For this review, take the finished solid that the model builds, in its own axes (mm). A direction names the side the tool comes from. Coordinates: 2 decimals unless noted, no trailing zeros. Write each loop counter-clockwise with the first axis right and the second up, starting at its lowest first coordinate (ties: lowest second). Pieces come first, ordered by that corner, then holes.
1) Insertion check: P1, Ø5.5, axis at y = 8, z = 6.5, coming from the +X side; P2, Ø3, axis at x = 2, y = -10.5, coming from the -Z side; P3, Ø4, axis at x = 0.5, y = 6.5, coming from the -Z side; P4, Ø1.5, axis at y = 6, z = 8, coming from the -X side. Each pin has a flat end and moves straight along its axis. Give the tip position at first contact, or say it passes through.
2) Mouldability with a two-part tool opening along X and no side actions: class faces 1 (the face through (-1.35, -9, 9)), 2 (the face through (0.942, 2.272, 4.052)), 3 (the face through (0.02, -6.2, 10.37)), 4 (the face through (4.506, -0.082, 3.944)) as pulls with the +X half, pulls with the -X half, needs draft (parallel to the pull), parting line crosses it, or undercut.
3) To check wall thickness, follow line 1 along Y through (x, z) = (0, 2.25); line 2 along Y through (x, z) = (1, 10.75); line 3 along X through (y, z) = (8.5, 13). State the ranges of each line that lie inside material, in increasing order.
4) We need section D-D on z = 2.25. Write out the cut boundary in (x, y), then the cut area to 3 significant figures.
5) We need section A-A on y = 0. Write out the cut boundary in (x, z), then the cut area to 3 significant figures.
6) We need section C-C on z = 10.25. Write out the cut boundary in (x, y), then the cut area to 3 significant figures.
7) For faces 5 (the face through (-3, -1, 8)), 6 (the face through (-0.02, 13.49, 14.13)), list the 3-axis set-ups (+Z, -Z, +X, -X, +Y, -Y) from which the entire face can be reached by the end or side of a thin tool; tool diameter is ignored.
from build123d import *

# Parameters (mm, degrees)
PAD_DEPTH = 1.35


with BuildPart() as pad:
    # Sketch001 → Pad (new body, symmetric)
    with BuildSketch(Plane.YZ):
        with BuildLine():
            Line((3, 0), (3, 8))
            Line((3, 8), (5, 8))
            Line((5, 8), (7.430632, 12.805439))
            ThreePointArc((13.716382, 8.063801), (13.408875, 14.193324), (7.430632, 12.805439))
            Line((5, 0), (13.716382, 8.063801))
            Line((3, 0), (5, 0))
        make_face()
        with BuildLine():
            Line((-13.716382, 8.063801), (-5, 0))
            Line((-5, 0), (-3, 0))
            Line((-3, 0), (-3, 8))
            Line((-3, 8), (-5, 8))
            Line((-5, 8), (-7.430632, 12.805439))
            ThreePointArc((-7.430632, 12.805439), (-13.408875, 14.193324), (-13.716382, 8.063801))
        make_face()
    extrude(amount=PAD_DEPTH, both=True)


with BuildPart() as obj1:
    # Sketch → Revolution (revolve)
    with BuildSketch(Plane.YZ):
        Polygon((3, 0), (2.46, 0.311769), (2.46, 7.688231), (3, 8), (4, 8), (5, 0), align=None)
    revolve(axis=Axis((0, 0, 0), (0, 0, 1)))

    # Fusion: union Pad
    add(pad.part)


solid = obj1.part
Result:
1. P1: stops at x = 1.35
1. P2: stops at z = 3.84
1. P3: stops at z = 0
1. P4: stops at x = -1.35
2. face 1: pulls with the -X half
2. face 2: undercut
2. face 3: needs draft
2. face 4: pulls with the +X half
3. line 1: y = -7.43 to -2.46, 2.46 to 7.43
3. line 2: y = -14.99 to -6.39, 6.39 to 14.99
3. line 3: x = -1.35 to 1.35
4. outline: (-1.35, -7.43) - (1.35, -7.43) - (1.35, -4.52) arc R4.72 ccw to (1.35, 4.52) - (1.35, 7.43) - (-1.35, 7.43) - (-1.35, 4.52) arc R4.72 ccw to (-1.35, -4.52) - close; hole circle Ø4.92 at (0, 0)
4. area: 65.9 mm2
5. outline: (-5, 0) - (-3, 0) - (-2.46, 0.31) - (-2.46, 7.69) - (-3, 8) - (-4, 8) - close; (2.46, 0.31) - (3, 0) - (5, 0) - (4, 8) - (3, 8) - (2.46, 7.69) - close
5. area: 32.3 mm2
6. outline: (-1.35, -14.93) - (1.35, -14.93) - (1.35, -6.14) - (-1.35, -6.14) - close; (-1.35, 6.14) - (1.35, 6.14) - (1.35, 14.93) - (-1.35, 14.93) - close
6. area: 47.5 mm2
7. face 5: +Z, +X, -X
7. face 6: +X, -X
